from build123d import *

# Parameters (mm, degrees)
SKETCH1_R           = 2.4892
BOSS_EXTRUDE1_DEPTH = 11.1125
FILLET1_R           = 1.5875
CUT_EXTRUDE1_DEPTH  = 5.08
SKETCH4_W           = 15.875
SKETCH4_H           = 19.05
CUT_EXTRUDE2_DEPTH  = 2.54
SKETCH5_R           = 2.4892
CUT_EXTRUDE3_DEPTH  = 104.567416874
FILLET2_R           = 1.524
CUT_EXTRUDE4_DEPTH  = 4.7625


with BuildPart() as part:
    # Sketch1 → Boss-Extrude1 (new, symmetric)
    with BuildSketch(Plane(origin=(0, 0, 0), x_dir=(0, 0, -1), z_dir=(1, 0, 0))):
        with BuildLine():
            Line((-9.525, 2.5527), (-9.525, -25.4))
            ThreePointArc((-9.525, -25.4), (-8.519418994, -29.659709497), (-5.715, -33.02))
            Line((-5.715, -33.02), (9.525, -44.45))
            Line((9.525, -44.45), (9.525, 6.116314701))
            ThreePointArc((9.525, 6.116314701), (3.528372392, 19.99118296), (-10.686230362, 25.130889218))
            Line((-10.686230362, 25.130889218), (-94.646476787, 20.003391506))
            ThreePointArc((-94.646476787, 20.003391506), (-100.60644719, 13.471571567), (-94.2594, 7.3152))
            Line((-94.2594, 7.3152), (-14.2875, 7.3152))
            ThreePointArc((-14.2875, 7.3152), (-10.919903955, 5.920296045), (-9.525, 2.5527))
        make_face()
        Circle(SKETCH1_R, mode=Mode.SUBTRACT)
        with Locations((0, -25.4)):
            Circle(SKETCH1_R, mode=Mode.SUBTRACT)
    extrude(amount=BOSS_EXTRUDE1_DEPTH, both=True)

    # Fillet1
    fillet1_edges = [part.edges().sort_by_distance(p)[0] for p in [
        (0, -44.45, -9.525),
    ]]
    fillet(fillet1_edges, radius=FILLET1_R)

    # Sketch3 → Cut-Extrude1 (cut)
    with BuildSketch(Plane.ZY.offset(11.1125)):
        Polygon((0, 7.332348419), (-6.35, 3.666174209), (-6.35, -3.666174209), (0, -7.332348419), (6.35, -3.666174209), (6.35, 3.666174209), align=None)
        Polygon((0, -18.067651581), (-6.35, -21.733825791), (-6.35, -29.066174209), (0, -32.732348419), (6.35, -29.066174209), (6.35, -21.733825791), align=None)
    cut_extrude1 = extrude(amount=-CUT_EXTRUDE1_DEPTH, mode=Mode.SUBTRACT)

    # Mirror1: Cut-Extrude1 across plane
    add(cut_extrude1.mirror(Plane(origin=(0, 0, 0), x_dir=(0, 0, 1), z_dir=(1, 0, 0))), mode=Mode.SUBTRACT)

    # Sketch4 → Cut-Extrude2 (cut)
    with BuildSketch(Plane.XY.offset(9.525)):
        with Locations((0, -12.7)):
            Rectangle(SKETCH4_W, SKETCH4_H)
    extrude(amount=-CUT_EXTRUDE2_DEPTH, mode=Mode.SUBTRACT)

    # Sketch5 → Cut-Extrude3 (cut, through all)
    with BuildSketch(Plane.XY.offset(6.985)):
        with Locations((0, -12.7)):
            Circle(SKETCH5_R)
    extrude(amount=-CUT_EXTRUDE3_DEPTH, mode=Mode.SUBTRACT)

    # Fillet2
    fillet2_edges = [part.edges().sort_by_distance(p)[0] for p in [
        (-11.1125, 22.567140362, 52.666353575),
        (-11.1125, 19.99118296, -3.528372392),
        (-11.1125, -37.7825, -0.635),
        (-11.1125, -29.659709497, 8.519418994),
        (11.1125, 19.99118296, -3.528372392),
        (11.1125, 22.567140362, 52.666353575),
        (11.1125, 13.471571567, 100.60644719),
        (11.1125, 7.3152, 54.27345),
        (11.1125, 5.920296045, 10.919903955),
        (11.1125, -11.42365, 9.525),
        (-11.1125, -17.579342649, -9.525),
        (11.1125, -17.579342649, -9.525),
        (-11.1125, -42.694903166, -8.647451583),
        (11.1125, -42.694903166, -8.647451583),
        (11.1125, -29.659709497, 8.519418994),
        (11.1125, -37.7825, -0.635),
        (-11.1125, -11.42365, 9.525),
        (-11.1125, 5.920296045, 10.919903955),
        (-11.1125, 7.3152, 54.27345),
        (-11.1125, 13.471571567, 100.60644719),
    ]]
    fillet(fillet2_edges, radius=FILLET2_R)

    # Sketch6 → Cut-Extrude4 (cut)
    with BuildSketch(Plane(origin=(0, 0, -9.525), x_dir=(-1, 0, 0), z_dir=(0, 0, -1))):
        Polygon((0, -18.199261314), (4.7625, -15.449630657), (4.7625, -9.950369343), (0, -7.200738686), (-4.7625, -9.950369343), (-4.7625, -15.449630657), align=None)
    extrude(amount=-CUT_EXTRUDE4_DEPTH, mode=Mode.SUBTRACT)


solid = part.part
Here's how the part is built. I have some questions about the finished solid (model axes, mm). A direction names the side the tool comes from. Coordinates: 2 decimals unless noted, no trailing zeros. Write each loop counter-clockwise with the first axis right and the second up, starting at its lowest first coordinate (ties: lowest second). Pieces come first, ordered by that corner, then holes.
Item 1: Will these pins go through, and if not, where does the flat tip stop? pin 1 (2 mm diameter, centred on x = -4, z = 8, fed in from -Y); pin 2 (5.5 mm diameter, centred on y = -25.4, z = 0, fed in from +X); pin 3 (6 mm diameter, centred on x = 7, z = 78, fed in from +Y).
Item 2: On a 3-axis mill with a long thin cutter (end or side, diameter ignored), from which of +Z, -Z, +X, -X, +Y, -Y can I reach the whole of each face in a straight line? I mean faces 1 (the cylindrical face through (0.13, 13.61, 100.61)), 2 (the flat face through (2.41, -16.81, -7.18)), 3 (the flat face through (0, -3.175, 8)), 4 (the flat face through (-8.608, 5.525, -3.131)), 5 (the flat face through (8.608, -19.926, 3.219)). Say none if no direction works.
Item 3: I want a section at B-B on y = -12.7. Write out the boundary of the cut face in (x, z) (1 decimal).
Item 4: If I drill on line 1 (Z direction, x = -2.5, y = -25.4) (3 decimals); line 2 (Y direction, x = 1, z = 0); line 3 (Y direction, x = 0, z = 0.5), over which ranges is the centre line in solid material (lowest first)?
Item 5: If we mould it in two halves opening along X, with no side actions, what happens to faces 6 (the flat face through (2, -10, 6.985)), 7 (the flat face through (-11.112, 11, 34)), 8 (the flat face through (0.1, 22.6, 52.1)), 9 (the cylindrical face through (1.34, -10.6, 1.19))? For each: +X half, -X half, draft (parallel to the pull), parting line (faces both ways), or undercut.
Findings below:
1. pin 1: stops at y = -31.86
1. pin 2: stops at x = 6.03
1. pin 3: stops at y = 21.2
2. face 1: +Z, +X, -X
2. face 2: -Z
2. face 3: +Z
2. face 4: -X
2. face 5: +X
3. outline: (-11.1, -8) arc R1.5 ccw to (-9.6, -9.5) - (-4.8, -9.5) - (-4.8, -4.8) - (-2.5, -4.8) - (-2.5, 7) - (-7.9, 7) - (-7.9, 9.5) - (-9.6, 9.5) arc R1.5 ccw to (-11.1, 8) - close; (2.5, -4.8) - (4.8, -4.8) - (4.8, -9.5) - (9.6, -9.5) arc R1.5 ccw to (11.1, -8) - (11.1, 8) arc R1.5 ccw to (9.6, 9.5) - (7.9, 9.5) - (7.9, 7) - (2.5, 7) - close
4. line 1: z = -9.525 to -2.489, 2.489 to 9.525
4. line 2: y = -37.31 to -27.89, -22.91 to -14.98, -10.42 to -2.49, 2.49 to 22.61
4. line 3: y = -36.93 to -27.84, -22.96 to -15.19, -10.21 to -2.44, 2.44 to 22.89
5. face 6: undercut
5. face 7: -X half
5. face 8: draft
5. face 9: undercut
